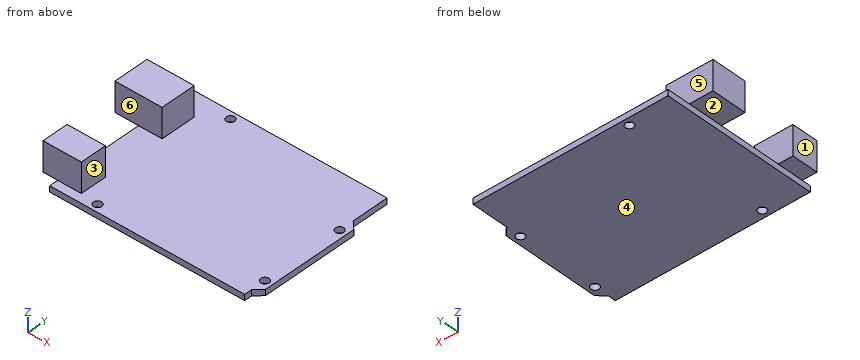
```python
from build123d import *

# Parameters (mm, degrees)
F0_R     = 1.4
F1_DEPTH = 2
F2_W     = 8
F2_H     = 12
F2_W_2   = 5
F2_H_2   = 9
F3_DEPTH = 10


with BuildPart() as f1:
    # F0 (on Top) → F1 (new body)
    with BuildSketch(Plane.XY):
        Polygon((86.1, 63.2), (20, 63.2), (20, 10), (86.1, 10), (86.1, 12.55), (88.6, 15.05), (88.6, 48.05), (86.1, 50.55), align=None)
        with Locations((34, 12.5)):
            Circle(F0_R, mode=Mode.SUBTRACT)
        with Locations((86.1, 17.6)):
            Circle(F0_R, mode=Mode.SUBTRACT)
        with Locations((35.3, 60.7)):
            Circle(F0_R, mode=Mode.SUBTRACT)
        with Locations((86.1, 45.5)):
            Circle(F0_R, mode=Mode.SUBTRACT)
    extrude(amount=F1_DEPTH)

    # F2 (on face) → F3 (join)
    with BuildSketch(Plane.XY.offset(2)):
        with Locations((16, 49.2)):
            Rectangle(F2_W, F2_H)
        with Locations((24, 49.2)):
            Rectangle(F2_W, F2_H)
        with Locations((17.5, 17.5)):
            Rectangle(F2_W_2, F2_H_2)
        with Locations((24, 17.5)):
            Rectangle(F2_W, F2_H_2)
    extrude(amount=F3_DEPTH)


solid = f1.part
```
For this review, take the finished solid that the model builds, in its own axes (mm). Face numbers are marked on the shaded views. A direction names the side the tool comes from. Round coordinates to 2 decimals unless told otherwise and drop trailing zeros. Write each loop counter-clockwise with the first axis right and the second up, starting at its lowest first coordinate (ties: lowest second). Pieces come first, ordered by that corner, then holes. Notation, with made-up numbers: (3.5, -10) - (13.5, -10) arc R18 cw to (13.5, -5) - close; hole circle Ø9 at (52.5, 8.5). An arc over 180 degrees is marked (long way). Answer as CSV lines item,"result". Start each with the question number.
(1) Add section A-A, the plane y = 17.6. State the section outline as (x, z) points.
(2) For line 1 (Y direction, x = 20.5, z = 5); line 2 (X direction, y = 19, z = 4.5); line 3 (Z direction, x = 61, y = 55), list the stretches that pass through material, from the lowest coordinate up.
(3) For pin 1 (0.6 mm diameter, centred on y = 55, z = 1, fed in from +X); pin 2 (7 mm diameter, centred on y = 17, z = 5, fed in from -X); pin 3 (1 mm diameter, centred on y = 31, z = 1.5, fed in from -X), all flat-tipped, find the tip position at first contact; note any pin that passes through.
(4) Machinability: for the marked faces 1, 2 and 3, which of the approach directions +Z, -Z, +X, -X, +Y, -Y give a long, thin tool a straight path to every point of the face, cutting with its end or side? Answer none if there is none.
(5) Add section B-B, the plane z = 3.25. State the section outline as (x, y) points, plus the area to 3 significant figures.
(6) Add section D-D, the plane x = 71.5. State the section outline as (y, z) points, plus the area to 3 significant figures.
(7) Mouldability with a two-part tool opening along Y and no side actions: class the marked faces 4, 5 and 6 as +Y half, -Y half, draft (parallel to the pull), parting line (faces both ways), or undercut.
(8) Add section C-C, the plane y = 60.7. State the section outline as (x, z) points, plus the area to 3 significant figures.
From the geometry:
1,outline,"(15, 2) - (20, 2) - (20, 0) - (84.7, 0) - (84.7, 2) - (28, 2) - (28, 12) - (15, 12) - close; (87.5, 0) - (88.6, 0) - (88.6, 2) - (87.5, 2) - close"
2,line 1,"y = 13 to 22, 43.2 to 55.2"
2,line 2,"x = 15 to 28"
2,line 3,"z = 0 to 2"
3,pin 1,"stops at x = 86.1"
3,pin 2,"stops at x = 15"
3,pin 3,"stops at x = 20"
4,face 1,"+Z, -Z, -X, -Y"
4,face 2,"-Z, -X, +Y, -Y"
4,face 3,"+Z, +X, +Y, -Y"
5,outline,"(12, 43.2) - (28, 43.2) - (28, 55.2) - (12, 55.2) - close; (15, 13) - (28, 13) - (28, 22) - (15, 22) - close"
5,area,"309 mm²"
6,outline,"(10, 0) - (63.2, 0) - (63.2, 2) - (10, 2) - close"
6,area,"106 mm²"
7,face 4,"draft"
7,face 5,"+Y half"
7,face 6,"undercut"
8,outline,"(20, 0) - (33.9, 0) - (33.9, 2) - (20, 2) - close; (36.7, 0) - (86.1, 0) - (86.1, 2) - (36.7, 2) - close"
8,area,"127 mm²"
